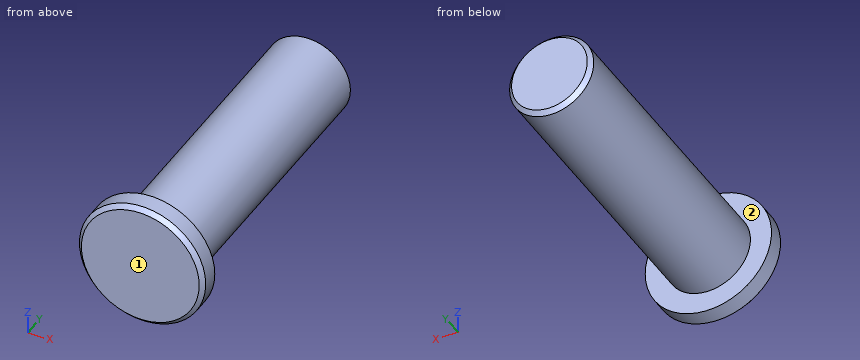
```python
from build123d import *

# Parameters (mm, degrees)
SKETCH_1_R      = 15
EXTRUDE_1_DEPTH = 5
SKETCH_2_R      = 10
EXTRUDE_2_DEPTH = 70
CHAMFER_1_SIZE  = 1


with BuildPart() as part:
    # 草图1 → 凸台-拉伸1 (new body)
    with BuildSketch(Plane(origin=(0, 0, 0), x_dir=(1, 0, 0), z_dir=(0, 1, 0))):
        Circle(SKETCH_1_R)
    extrude(amount=EXTRUDE_1_DEPTH)

    # 草图2 → 凸台-拉伸2 (add)
    with BuildSketch(Plane(origin=(0, 5, 0), x_dir=(1, 0, 0), z_dir=(0, 1, 0))):
        Circle(SKETCH_2_R)
    extrude(amount=EXTRUDE_2_DEPTH)

    # 倒角1
    chamfer_1_edges = [part.edges().sort_by_distance(p)[0] for p in [
        (-15, 0, 0),
        (-10, 75, 0),
    ]]
    chamfer(chamfer_1_edges, length=CHAMFER_1_SIZE)


solid = part.part
```
Input: part model. Units: mm. Frame: model coordinates. Face numbers are marked on the shaded views. A direction names the side the tool comes from. Round coordinates to 2 decimals unless told otherwise and drop trailing zeros. Loops run counter-clockwise (first coordinate to the right, second up) from the corner with the lowest first, then second, coordinate; pieces in that order, holes last. Notation, with made-up numbers: (0.5, 18.5) - (47.5, 18.5) arc R19 cw to (47.5, 46.5) - close; hole circle Ø3 at (-22.75, -26). An arc over 180 degrees is marked (long way). One line per item, written item: value. Start each with the question number.
(1) Section B-B, the plane x = 0. Return loops of the section in (y, z).
(2) Ray query, line 1 (Y direction, x = 3.75, z = 13.5); line 2 (Z direction, x = 0.25, y = 44). Return the intervals inside material, ascending. Write a range as [from, to].
(3) Section C-C, the plane y = 14. Return loops of the section in (x, z), plus the area to 3 significant figures.
(4) Access query for the marked faces 1 and 2. Directions: +Z, -Z, +X, -X, +Y, -Y. A direction counts if a zero-diameter tool reaches every point of the face in a straight line with its end or side. Return the directions, or none.
(5) Section A-A, the plane z = 0. Return loops of the section in (x, y), plus the area to 3 significant figures.
(6) Contact query for flat-ended pins moving along their axis: P1, Ø4, axis at x = 1.5, y = 50, coming from the +Z side; P2, Ø1, axis at x = 4.5, y = 8.5, coming from the -Z side; P3, Ø1.5, axis at y = 36.5, z = -4.5, coming from the +X side; P4, Ø12, axis at x = -6.5, z = 11.5, coming from the -Y side. Output: stop coordinate, or through.
Results below:
1. outline: (0, -14) - (1, -15) - (5, -15) - (5, -10) - (74, -10) - (75, -9) - (75, 9) - (74, 10) - (5, 10) - (5, 15) - (1, 15) - (0, 14) - close
2. line 1: [0.01, 5]
2. line 2: [-10, 10]
3. outline: circle Ø20 at (0, 0)
3. area: 314 mm^2
4. face 1: +Z, -Z, +X, -X, -Y
4. face 2: +Y
5. outline: (-15, 1) - (-14, 0) - (14, 0) - (15, 1) - (15, 5) - (10, 5) - (10, 74) - (9, 75) - (-9, 75) - (-10, 74) - (-10, 5) - (-15, 5) - close
5. area: 1,550 mm^2
6. P1: z = 10
6. P2: z = -9.17
6. P3: x = 9.27
6. P4: y = 0
